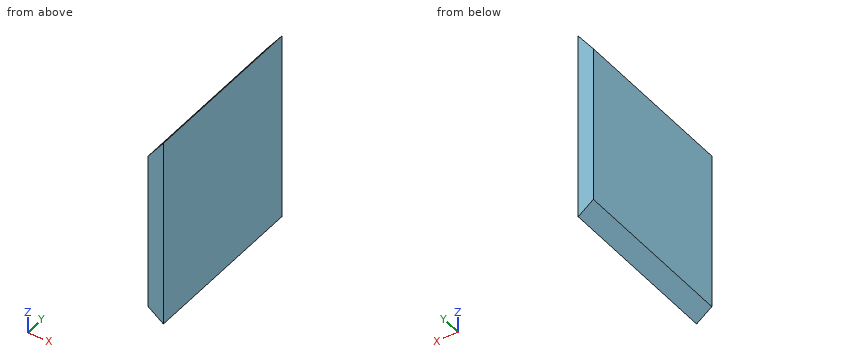
from build123d import *

# Parameters (mm, degrees)
SKETCH1_W           = 75
SKETCH1_H           = 68
BOSS_EXTRUDE1_DEPTH = 6
CUT_EXTRUDE1_DEPTH  = 78.886134838
CUT_EXTRUDE2_DEPTH  = 78.886134838


with BuildPart() as part:
    # Sketch1 → Boss-Extrude1 (new body)
    with BuildSketch(Plane(origin=(0, 0, 0), x_dir=(0, 0, -1), z_dir=(1, 0, 0))):
        Rectangle(SKETCH1_W, SKETCH1_H)
    extrude(amount=BOSS_EXTRUDE1_DEPTH)

    # Sketch2 → Cut-Extrude1 (cut, through all)
    with BuildSketch(Plane(origin=(0, 34, 0), x_dir=(1, 0, 0), z_dir=(0, 1, 0))):
        Polygon((6, 37.5), (0, 33), (0, 37.5), align=None)
    extrude(amount=-CUT_EXTRUDE1_DEPTH, mode=Mode.SUBTRACT)

    # Sketch3 → Cut-Extrude2 (cut, through all)
    with BuildSketch(Plane(origin=(0, 34, 0), x_dir=(1, 0, 0), z_dir=(0, 1, 0))):
        Polygon((6, -37.5), (0, -29.5), (0, -37.5), align=None)
    extrude(amount=-CUT_EXTRUDE2_DEPTH, mode=Mode.SUBTRACT)


solid = part.part
Check sheet for the modelled part. Datum: model origin and axes. Units: mm. Round coordinates to 2 decimals unless told otherwise and drop trailing zeros. Order: outer loops, then holes, each group sorted by start corner. A loop starts at its lowest first (then second) coordinate and runs counter-clockwise, first axis right, second up.
Q1. Scan lines: L1, parallel to Z at x = 1.25, y = -17; L2, parallel to Z at x = 1.75, y = 17; L3, parallel to X at y = 24.5, z = 32.5. Record each from-to range of solid material in increasing order.
Filled sheet:
L1: z = -33.94 to 31.17
L2: z = -34.31 to 31.83
L3: x = 2.25 to 6
Q2. Cross-section at A-A, the plane x = 3. Enter the section's corners in (y, z), plus the area to 4 significant figures.
Filled sheet:
outline: (-34, -35.25) - (34, -35.25) - (34, 33.5) - (-34, 33.5) - close
area: 4,675 mm2
Q3. Cross-section at B-B, the plane y = 0.5. Enter the section's corners in (x, z), plus the area to 4 significant figures.
Filled sheet:
outline: (0, -33) - (6, -37.5) - (6, 37.5) - (0, 29.5) - close
area: 412.5 mm2
Q4. Depth check by flat-ended pin: P1, Ø1.5, axis at x = 5.5, y = -5, coming from the +Z side. Enter the tip coordinate at first touch or a pass-through.
Filled sheet:
P1: stops at z = 37.5
